CAD build for the part. Positions are in the model's coordinates, mm. Give positions to 0.01 mm unless a question says otherwise; leave off trailing zeros. Order: outer loops, then holes, each group sorted by start corner. A loop starts at its lowest first (then second) coordinate and runs counter-clockwise, first axis right, second up. Notation, with made-up numbers: (5, 56) -> (57, 56) arc R37 ccw to (57, 94) -> close; hole circle Ø1 at (31, 34.5). An arc over 180 degrees is marked (long way). Answer as CSV lines item,"result".
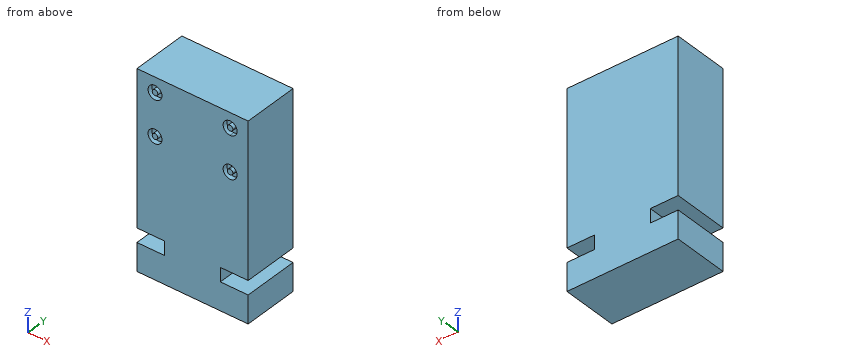
```python
from build123d import *

# Parameters (mm, degrees)
F1_DEPTH = 25.4
F2_R     = 3.175
F2_R_2   = 1.27
F3_DEPTH = 2.1166666667


with BuildPart() as f1:
    # F0 (on Front) → F1 (new body)
    with BuildSketch(Plane.XZ):
        Polygon((50.8, 0), (0, 0), (0, -69.85), (12.7, -69.85), (12.7, -76.2), (0, -76.2), (0, -88.9), (50.8, -88.9), (50.8, -76.2), (38.1, -76.2), (38.1, -69.85), (50.8, -69.85), align=None)
    extrude(amount=-F1_DEPTH)

    # F2 (on face) → F3 (cut)
    with BuildSketch(Plane.XZ):
        with BuildLine():
            ThreePointArc((11.43, -6.82625), (8.255, -3.65125), (5.08, -6.82625))
            ThreePointArc((5.08, -6.82625), (8.255, -10.00125), (11.43, -6.82625))
        make_face()
        with BuildLine():
            ThreePointArc((6.985, -6.82625), (8.255, -5.55625), (9.525, -6.82625))
            ThreePointArc((9.525, -6.82625), (8.255, -8.09625), (6.985, -6.82625))
        make_face(mode=Mode.SUBTRACT)
        with BuildLine():
            Line((45.72, -6.82625), (43.815, -6.82625))
            ThreePointArc((43.815, -6.82625), (43.4430256121, -7.7242756121), (42.545, -8.09625))
            Line((42.545, -8.09625), (42.545, -10.00125))
            ThreePointArc((42.545, -10.00125), (44.7900640303, -9.0713140303), (45.72, -6.82625))
        make_face()
        with BuildLine():
            ThreePointArc((42.545, -8.09625), (41.6469743879, -5.9282243879), (43.815, -6.82625))
            Line((43.815, -6.82625), (45.72, -6.82625))
            ThreePointArc((45.72, -6.82625), (40.2999359697, -4.5811859697), (42.545, -10.00125))
            Line((42.545, -10.00125), (42.545, -8.09625))
        make_face()
        with BuildLine():
            ThreePointArc((45.72, -26.035), (44.7900640303, -23.7899359697), (42.545, -22.86))
            ThreePointArc((42.545, -22.86), (40.2999359697, -28.2800640303), (45.72, -26.035))
        make_face()
        with BuildLine():
            ThreePointArc((43.815, -26.035), (41.6469743879, -26.9330256121), (42.545, -24.765))
            ThreePointArc((42.545, -24.765), (43.4430256121, -25.1369743879), (43.815, -26.035))
        make_face(mode=Mode.SUBTRACT)
        with Locations((8.255, -26.035)):
            Circle(F2_R)
        with Locations((8.255, -26.035)):
            Circle(F2_R_2, mode=Mode.SUBTRACT)
    extrude(amount=-F3_DEPTH, mode=Mode.SUBTRACT)


solid = f1.part
```
1) Band-saw the part on A-A, the plane x = 3.5. Write the cut outline in (y, z).
Data:
outline,"(0, -88.9) -> (25.4, -88.9) -> (25.4, -76.2) -> (0, -76.2) -> close; (0, -69.85) -> (25.4, -69.85) -> (25.4, 0) -> (0, 0) -> close"
2) Pin check, flat tip, straight feed: P1, Ø5, axis at y = 10, z = -73.5, coming from the -X side. Stop position of the tip, or through.
Data:
P1,"stops at x = 12.7"
3) Wall check: line 1 along Z through (x, y) = (3, 18.5). Give the ranges that are in metal, low to high. Write a range as [from, to].
Data:
line 1,"z = [-88.9, -76.2], [-69.85, 0]"
4) Band-saw the part on C-C, the plane z = -73. Write the cut outline in (x, y).
Data:
outline,"(12.7, 0) -> (38.1, 0) -> (38.1, 25.4) -> (12.7, 25.4) -> close"
5) Band-saw the part on B-B, the plane y = 12.25. Write the cut outline in (x, z), then the cut area to 3 significant figures.
Data:
outline,"(0, -88.9) -> (50.8, -88.9) -> (50.8, -76.2) -> (38.1, -76.2) -> (38.1, -69.85) -> (50.8, -69.85) -> (50.8, 0) -> (0, 0) -> (0, -69.85) -> (12.7, -69.85) -> (12.7, -76.2) -> (0, -76.2) -> close"
area,"4,350 mm2"
